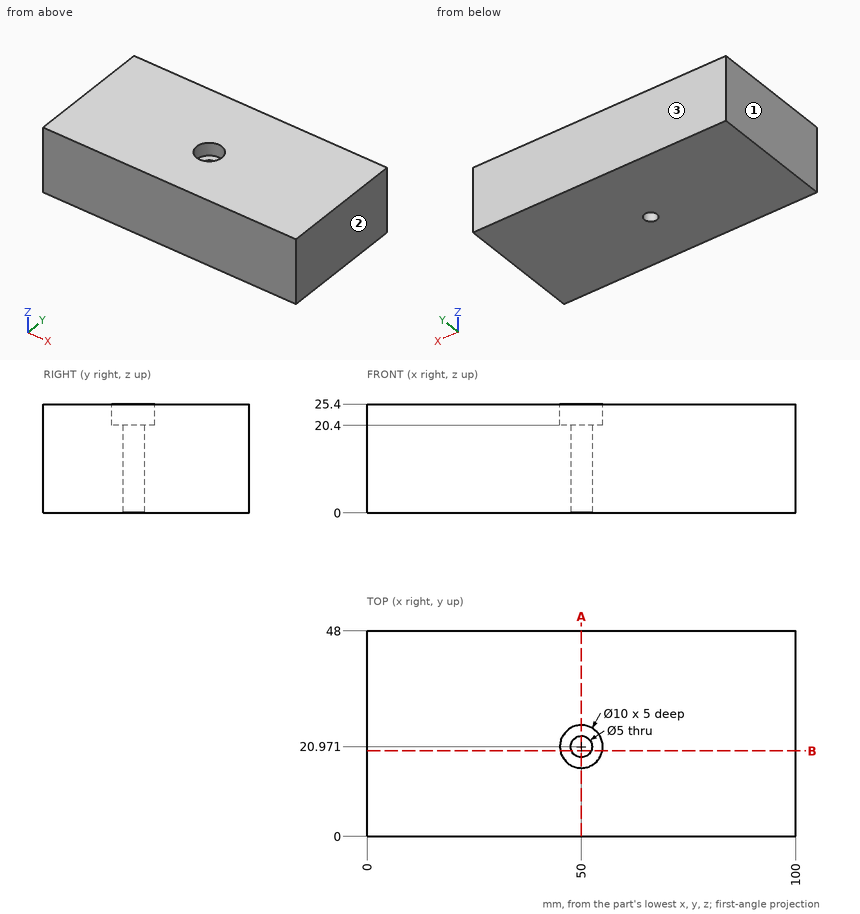
Answer from the drawing. Dimensions are ordinates in mm from the lowest x, y and z of the part. Give positions to 0.01 mm unless a question says otherwise; leave off trailing zeros. Order: outer loops, then holes, each group sorted by start corner. A loop starts at its lowest first (then second) coordinate and runs counter-clockwise, first axis right, second up. Notation, with made-up numbers: (20.5, -2.75) - (45.5, -2.75) arc R34 cw to (45.5, 33.25) - close; hole circle Ø3 at (18.25, 58). An arc over 180 degrees is marked (long way). One line per item, written item: value. Start each with the question number.
1. Consider line 1 (Y direction, x = 50, z = 10); line 2 (Y direction, x = 50, z = 22.9); line 3 (X direction, y = 21.5, z = 7.75). Determine where each line is inside the solid, lowest interval first.
2. Section B-B, the plane y = 20 is taken. Write down the section's boundary in (x, z) (1 decimal), then the cut area to 3 significant figures.
3. This flat-tipped pin is pushed along its axis until it touches: pin 1 Ø3 at (x, y) = (50, 20.97) entering from +Z. Where does it stop, or does it pass through?
4. Section A-A, the plane x = 50 is taken. Write down the section's boundary in (y, z), then the cut area to 3 significant figures.
5. For a pull along X with two mould halves and no side action, classify the marked faces 1, 2 and 3 as released by +X, released by -X, zero draft, split by the parting line, or undercut.
Filled sheet:
1. line 1: 0 to 18.47, 23.47 to 48
1. line 2: 0 to 15.97, 25.97 to 48
1. line 3: 0 to 47.56, 52.44 to 100
2. outline: (0, 0) - (47.7, 0) - (47.7, 20.4) - (45.1, 20.4) - (45.1, 25.4) - (0, 25.4) - close; (52.3, 0) - (100, 0) - (100, 25.4) - (54.9, 25.4) - (54.9, 20.4) - (52.3, 20.4) - close
2. area: 2,400 mm²
3. pin 1: through
4. outline: (0, 0) - (18.47, 0) - (18.47, 20.4) - (15.97, 20.4) - (15.97, 25.4) - (0, 25.4) - close; (23.47, 0) - (48, 0) - (48, 25.4) - (25.97, 25.4) - (25.97, 20.4) - (23.47, 20.4) - close
4. area: 1,070 mm²
5. face 1: released by -X
5. face 2: released by +X
5. face 3: zero draft
